The listing builds one solid part. Answer for the finished solid, in the listing's coordinates (mm). Face numbers are marked on the shaded views. A direction names the side the tool comes from. Coordinates: 2 decimals unless noted, no trailing zeros. Order: outer loops, then holes, each group sorted by start corner. A loop starts at its lowest first (then second) coordinate and runs counter-clockwise, first axis right, second up. Notation, with made-up numbers: (44, 6) - (59, 6) arc R17 ccw to (59, 26) - close; hole circle Ø4 at (86.5, 61.5). An arc over 180 degrees is marked (long way). Use a Markdown table: item, result. Add a question column.
Item 1: The part is cut by section D-D, the plane x = 3. Give the vertices of the cut face in (y, z), then the cut area to 3 significant figures.
Item 2: Flat-ended cylindrical pins translate along their axes: P1, Ø3, axis at y = -9.5, z = -7, coming from the +X side; P2, Ø2.5, axis at x = -23, y = -16.5, coming from the -Z side; P3, Ø1.8, axis at x = 22, y = -17, coming from the +Z side; P4, Ø7, axis at y = -5, z = -7, coming from the -X side. Find the tip coordinate at first contact, or state that the pin passes through.
Item 3: For the marked faces 3 and 4, determine the directions among +Z, -Z, +X, -X, +Y, -Y from which every point of the face is accessible in a straight line to the end or side of a thin tool.
Item 4: The part is cut by section C-C, the plane x = -23. Give the vertices of the cut face in (y, z), then the cut area to 3 significant figures.
Item 5: Find the intervals of material crossed by line 1 along Y through (x, z) = (-23, -23.2); line 2 along X through (y, z) = (9.5, -13); line 3 along Z through (x, y) = (9, 19), in increasing order.
Item 6: The part is cut by section A-A, the plane y = -3.5. Give the vertices of the cut face in (x, z).
Item 7: The mould has two halves that part along X. Classify the marked faces 1 and 2: released by +X, released by -X, zero draft, split by the parting line, or undercut.
Item 8: The part is cut by section B-B, the plane z = -11.25. Give the vertices of the cut face in (x, y).
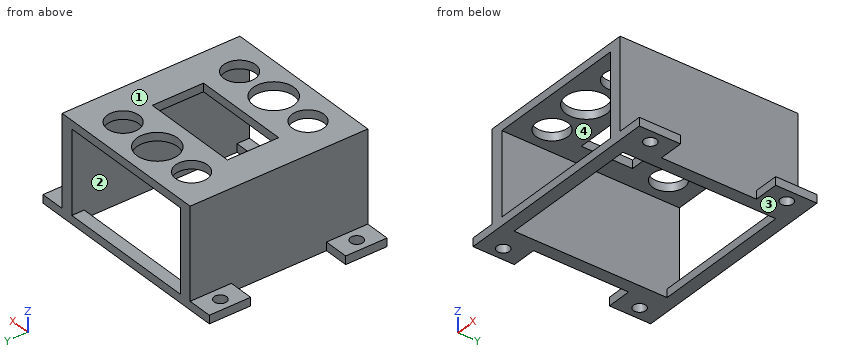
Autodesk Inventor part; units mm, degrees
ref_plane "Work Plane1" through (0, 0, -22) normal (0, 0, 1) x (1, 0, 0)
ref_plane "YZ Plane" through (0, 0, 0) normal (1, 0, 0) x (0, 1, 0)
ref_plane "XZ Plane" through (0, 0, 0) normal (0, 1, 0) x (-1, 0, 0)
sketch "Block1_1" plane through (0, 0, 0) normal (0, 0, 1) x (1, 0, 0)
  circle A0 centre (47.029, 24.2723) radius 1.1
  circle A1 centre (75.029, 24.2723) radius 1.1
  line L0 (49.279, 30.4723) -> (72.779, 30.4723)
  line L1 (72.779, 30.4723) -> (72.779, 18.0723)
  line L2 (72.779, 18.0723) -> (49.279, 18.0723)
  line L3 (49.279, 18.0723) -> (49.279, 30.4723)
  line L4 (49.279, 30.4723) -> (44.779, 30.4723)
  line L5 (44.779, 30.4723) -> (44.779, 18.0723)
  line L6 (44.779, 18.0723) -> (49.279, 18.0723)
  line L7 (49.279, 18.0723) -> (49.279, 30.4723)
  line L8 (72.779, 30.4723) -> (77.279, 30.4723)
  line L9 (77.279, 30.4723) -> (77.279, 18.0723)
  line L10 (77.279, 18.0723) -> (72.779, 18.0723)
  line L11 (72.779, 18.0723) -> (72.779, 30.4723)
  line L12 (44.779, 24.2723) -> (77.279, 24.2723) construction
  line L13 (61.029, 30.4723) -> (61.029, 18.0723) construction
  line L14 (47.029, 30.4723) -> (47.029, 18.0723) construction
  line L15 (75.029, 30.4723) -> (75.029, 18.0723) construction
  line L16 (66.779, 30.4723) -> (66.779, 18.0723) construction
  point P0 (60.979, 24.0984)
  dimension "d2" = 23.5
  dimension "d3" = 12.4
  dimension "d4" = 4.5
  dimension "d5" = 4.5
  dimension "d6" = 2.2
  dimension "d7" = 2.2
  dimension "d8" = 2.25
  dimension "d9" = 6
sketch "Sketch1" plane through (0, 0, 0) normal (0, 0, 1) x (1, 0, 0)
  line L0 (-20, 21.5) -> (20, 21.5)
  line L1 (20, 21.5) -> (20, -21.5)
  line L2 (20, -21.5) -> (-20, -21.5)
  line L3 (-20, -21.5) -> (-20, 21.5)
  line L4 (-0.1493, 33.2365) -> (-0.1493, -35.4112) construction
  line L5 (-27.052, 0) -> (29.4139, 0) construction
  line L6 (20, 21.5) -> (17, 21.5)
  line L7 (17, 21.5) -> (17, -21.5)
  line L8 (17, -21.5) -> (20, -21.5)
  line L9 (20, -21.5) -> (20, 21.5)
  line L10 (-20, 21.5) -> (-17, 21.5)
  line L11 (-17, 21.5) -> (-17, -21.5)
  line L12 (-17, -21.5) -> (-20, -21.5)
  line L13 (-20, -21.5) -> (-20, 21.5)
  line L14 (-20, 21.5) -> (20, 21.5)
  line L15 (20, 21.5) -> (20, -21.5)
  line L16 (20, -21.5) -> (-20, -21.5)
  line L17 (-20, -21.5) -> (-20, 21.5)
  circle A0 centre (-0.1493, 14.0909) radius 4.9337
  circle A1 centre (10.5202, 14.0909) radius 3.8489
  circle A2 centre (-10.8699, 14.0909) radius 3.8489
  circle A3 centre (-14.1493, 0) radius 1.1
  circle A4 centre (13.8507, 0) radius 1.1
  line L18 (-11.8993, 6.2) -> (11.6007, 6.2)
  line L19 (11.6007, 6.2) -> (11.6007, -6.2)
  line L20 (11.6007, -6.2) -> (-11.8993, -6.2)
  line L21 (-11.8993, -6.2) -> (-11.8993, 6.2)
  line L22 (-11.8993, 6.2) -> (-16.3993, 6.2)
  line L23 (-16.3993, 6.2) -> (-16.3993, -6.2)
  line L24 (-16.3993, -6.2) -> (-11.8993, -6.2)
  line L25 (-11.8993, -6.2) -> (-11.8993, 6.2)
  line L26 (11.6007, 6.2) -> (16.1007, 6.2)
  line L27 (16.1007, 6.2) -> (16.1007, -6.2)
  line L28 (16.1007, -6.2) -> (11.6007, -6.2)
  line L29 (11.6007, -6.2) -> (11.6007, 6.2)
  line L30 (-16.3993, 0) -> (16.1007, 0) construction
  line L31 (-0.1493, 6.2) -> (-0.1493, -6.2) construction
  line L32 (-14.1493, 6.2) -> (-14.1493, -6.2) construction
  line L33 (13.8507, 6.2) -> (13.8507, -6.2) construction
  line L34 (5.6007, 6.2) -> (5.6007, -6.2) construction
  point P0 (0, 0)
  point P1 (-20, 0)
  point P2 (0, -21.5)
  dimension "d0" = 40
  dimension "d1" = 43
  dimension "d10" = 3
  dimension "d11" = 3
extrude "Extrusion1" add sketch "Sketch1" against normal blind 2 contours L0 L7 L2 L11 | A0 | A1 | A2 | A3 | A4 | L21 L24 L23 L22 | L26 L27 L28 L19
extrude "Extrusion2" add sketch "Sketch1" against normal blind 22 contours L0 L11 L2 L3 | L0 L1 L2 L7
ref_plane "Work Plane1" through (0, 0, -22) normal (0, 0, 1) x (1, 0, 0)
sketch "Sketch2" plane through (0, 0, -22) normal (0, 0, 1) x (1, 0, 0)
  line L0 (-11.8993, 6.2) -> (11.6007, 6.2)
  line L1 (11.6007, -6.2) -> (-11.8993, -6.2)
  line L2 (20, 21.5) -> (-20, 21.5)
  line L3 (-20, 21.5) -> (-20, -21.5)
  line L4 (-20, -21.5) -> (20, -21.5)
  line L5 (20, -21.5) -> (20, 21.5)
  line L6 (-17, 18.5) -> (17, 18.5)
  line L7 (17, 18.5) -> (17, -18.5)
  line L8 (17, -18.5) -> (-17, -18.5)
  line L9 (-17, -18.5) -> (-17, 18.5)
  line L10 (20, 21.5) -> (26, 21.5)
  line L11 (26, 21.5) -> (26, 11.5)
  line L12 (26, 11.5) -> (20, 11.5)
  line L13 (20, 11.5) -> (20, 21.5)
  line L14 (20, -21.5) -> (26, -21.5)
  line L15 (26, -21.5) -> (26, -11.5)
  line L16 (26, -11.5) -> (20, -11.5)
  line L17 (20, -11.5) -> (20, -21.5)
  line L18 (-20, 21.5) -> (-26, 21.5)
  line L19 (-26, 21.5) -> (-26, 11.5)
  line L20 (-26, 11.5) -> (-20, 11.5)
  line L21 (-20, 11.5) -> (-20, 21.5)
  line L22 (-20, -21.5) -> (-26, -21.5)
  line L23 (-26, -21.5) -> (-26, -11.5)
  line L24 (-26, -11.5) -> (-20, -11.5)
  line L25 (-20, -11.5) -> (-20, -21.5)
  circle A0 centre (-23, 16.5) radius 1.5
  circle A1 centre (-23, -16.5) radius 1.5
  circle A2 centre (23, 16.5) radius 1.5
  circle A3 centre (23, -16.5) radius 1.5
  line L26 (-11.8993, -6.2) -> (-11.8993, 6.2)
  line L27 (11.6007, 6.2) -> (11.6007, -6.2)
  point P0 (0, 0)
  dimension "d17" = 3
  dimension "d22" = 6
  dimension "d23" = 10
  dimension "d24" = 6
  dimension "d25" = 10
  dimension "d26" = 6
  dimension "d27" = 10
  dimension "d28" = 6
  dimension "d29" = 10
  dimension "d30" = 3
  dimension "d31" = 3
  dimension "d32" = 3
  dimension "d33" = 3
extrude "Extrusion3" add sketch "Sketch2" against normal blind 2 contours L5 L4 L3 L2
extrude "Extrusion4" cut sketch "Sketch1" against normal blind 2 contours A0 | A1 | A2
mirror "Mirror1" about plane through (0, 0, 0) normal (0, 1, 0) of "Extrusion4"
extrude "Extrusion5" add sketch "Sketch2" against normal blind 2 contours L10 L11 L12 L5 | L3 L20 L19 L18 | L16 L15 L14 L5 | L3 L22 L23 L24
properties part number "ServoHolder"
Solution:
| question | item | result |
|---|---|---|
| 1 | outline | (-21.5, -24) - (-18.5, -24) - (-18.5, -22) - (-21.5, -22) - close; (-21.5, -2) - (-17.89, -2) - (-17.89, 0) - (-21.5, 0) - close; (-10.29, -2) - (-6.2, -2) - (-6.2, 0) - (-10.29, 0) - close; (6.2, -2) - (10.29, -2) - (10.29, 0) - (6.2, 0) - close; (17.89, -2) - (21.5, -2) - (21.5, 0) - (17.89, 0) - close; (18.5, -24) - (21.5, -24) - (21.5, -22) - (18.5, -22) - close |
| 1 | area | 42.8 mm2 |
| 2 | P1 | stops at x = 20 |
| 2 | P2 | passes through |
| 2 | P3 | stops at z = -22 |
| 2 | P4 | stops at x = -20 |
| 3 | face 3 | -Z, +X, -X, +Y, -Y |
| 3 | face 4 | +Y, -Y |
| 4 | outline | (-21.5, -24) - (-18, -24) - (-18, -22) - (-21.5, -22) - close; (-15, -24) - (-11.5, -24) - (-11.5, -22) - (-15, -22) - close; (11.5, -24) - (15, -24) - (15, -22) - (11.5, -22) - close; (18, -24) - (21.5, -24) - (21.5, -22) - (18, -22) - close |
| 4 | area | 28.0 mm2 |
| 5 | line 1 | y = -21.5 to -18, -15 to -11.5, 11.5 to 15, 18 to 21.5 |
| 5 | line 2 | x = -20 to -17, 17 to 20 |
| 5 | line 3 | z = -24 to -22, -2 to 0 |
| 6 | outline | (-20, -24) - (-17, -24) - (-17, -2) - (-11.9, -2) - (-11.9, 0) - (-20, 0) - close; (11.6, -2) - (17, -2) - (17, -24) - (20, -24) - (20, 0) - (11.6, 0) - close |
| 7 | face 1 | zero draft |
| 7 | face 2 | undercut |
| 8 | outline | (-20, -21.5) - (-17, -21.5) - (-17, 21.5) - (-20, 21.5) - close; (17, -21.5) - (20, -21.5) - (20, 21.5) - (17, 21.5) - close |
